Input: dimensioned drawing with shaded views. Units: mm. Origin: part minimum x, y, z. A direction names the side the tool comes from. Round coordinates to 2 decimals unless told otherwise and drop trailing zeros. Loops run counter-clockwise (first coordinate to the right, second up) from the corner with the lowest first, then second, coordinate; pieces in that order, holes last. Notation, with made-up numbers: M 61.25,59.25 L 113.25,59.25 A10 cw 113.25,76.25 Z; hole C -14,43 d2. An arc over 180 degrees is marked long. Use one line per item in the form item = value. Start each with the question number.
Q1. Ray query, line 1 along Z through (x, y) = (233, 20); line 2 along Y through (x, z) = (12, 20); line 3 along X through (y, z) = (85, 25). Return the intervals inside material, ascending.
Q2. Section query C-C, the plane x = 37.5. Output: boundary loops of the cut face in (y, z).
Q3. Mould query, pull axis Z, two halves, no side actions, for the marked faces 1, 2, 3 and 4. Classes: pulls with the +Z half, pulls with the -Z half, needs draft (parallel to the pull), parting line crosses it, or undercut.
Q4. Section query D-D, the plane x = 174. Output: boundary loops of the cut face in (y, z) (1 decimal).
Q5. First-contact query: P1, Ø22, axis at x = 62.5, y = 90.5, coming from the -Z side; P2, Ø6, axis at x = 140, z = 50.5, coming from the +Y side; P3, Ø12, axis at x = 181.5, z = 67, coming from the -Y side. Flat tips, straight axial feed; report the tip coordinate or a pass-through.
Q6. Access query for the marked faces 5, 6 and 7. Directions: +Z, -Z, +X, -X, +Y, -Y. A direction counts if a zero-diameter tool reaches every point of the face in a straight line with its end or side. Return the directions, or none.
Q7. Section query B-B, the plane x = 108. Output: boundary loops of the cut face in (y, z).
Q8. Section query A-A, the plane y = 57. Output: boundary loops of the cut face in (x, z) (1 decimal), and give its area (3 significant figures).
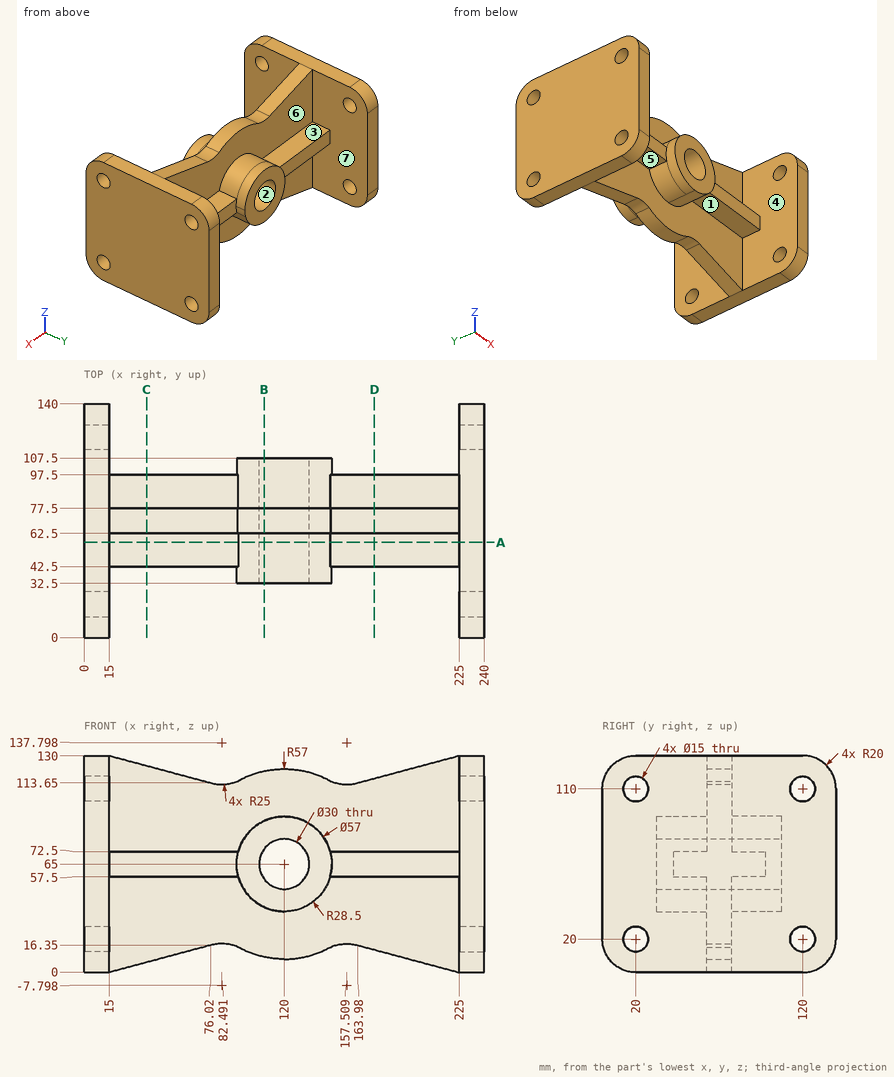
Results found:
q1.line_1 = 0 to 12.5, 27.5 to 102.5, 117.5 to 130
q1.line_2 = 0 to 12.5, 27.5 to 112.5, 127.5 to 140
q1.line_3 = 0 to 15, 225 to 240
q2.outline = M 42.5,57.5 L 62.5,57.5 L 62.5,6.03 L 77.5,6.03 L 77.5,57.5 L 97.5,57.5 L 97.5,72.5 L 77.5,72.5 L 77.5,123.97 L 62.5,123.97 L 62.5,72.5 L 42.5,72.5 Z
q3.face_1 = pulls with the -Z half
q3.face_2 = undercut
q3.face_3 = pulls with the +Z half
q3.face_4 = needs draft
q4.outline = M 42.5,57.5 L 62.5,57.5 L 62.5,13.7 L 77.5,13.7 L 77.5,57.5 L 97.5,57.5 L 97.5,72.5 L 77.5,72.5 L 77.5,116.3 L 62.5,116.3 L 62.5,72.5 L 42.5,72.5 Z
q5.P1 = 57.5
q5.P2 = 107.5
q5.P3 = 42.5
q6.face_5 = -Z, -Y
q6.face_6 = +Z, +Y
q6.face_7 = +Y
q7.outline = M 32.5,39.15 L 62.5,39.15 L 62.5,9.28 L 77.5,9.28 L 77.5,39.15 L 107.5,39.15 L 107.5,56 L 32.5,56 Z; M 32.5,74 L 107.5,74 L 107.5,90.85 L 77.5,90.85 L 77.5,120.72 L 62.5,120.72 L 62.5,90.85 L 32.5,90.85 Z
q8.outline = M 0,0 L 15,0 L 15,57.5 L 92.5,57.5 A28.5 ccw 147.5,57.5 L 225,57.5 L 225,0 L 240,0 L 240,130 L 225,130 L 225,72.5 L 147.5,72.5 A28.5 ccw 92.5,72.5 L 15,72.5 L 15,130 L 0,130 Z; hole C 120,65 d30
q8.area = 8,050 mm²
